Input: part model. Units: mm. Frame: model coordinates. Face numbers are marked on the shaded views. A direction names the side the tool comes from. Give positions to 0.01 mm unless a question says otherwise; leave off trailing zeros. Write each loop counter-clockwise with the first axis right and the second up, starting at its lowest first coordinate (ties: lowest second). Pieces come first, ordered by that corner, then holes. Notation, with made-up numbers: (40.5, 18.25) - (85.5, 18.25) arc R13 ccw to (85.5, 37.25) - close; hole circle Ø4 at (-27.5, 44.25). An arc over 180 degrees is marked (long way). Answer as CSV lines item,"result". Start each with the question number.
from build123d import *

# Parameters (mm, degrees)
BASE_FLANGE1_DEPTH = 15
SKETCH6_R          = 1.64265796
CUT_EXTRUDE1_DEPTH = 0.7


# Sheet-metal steps are written as plain solids
with BuildPart() as part:
    # Sketch1 → Base-Flange1 (new body)
    with BuildSketch(Plane.XY):
        with BuildLine():
            Line((0, 0), (59.3, 0))
            ThreePointArc((59.3, 0), (59.794974747, 0.205025253), (60, 0.7))
            Line((60, 0.7), (60, 73.6))
            ThreePointArc((60, 73.6), (60.410050506, 74.589949494), (61.4, 75))
            Line((61.4, 75), (150, 75))
            Line((150, 75), (150, 74.3))
            Line((150, 74.3), (61.4, 74.3))
            ThreePointArc((61.4, 74.3), (60.905025253, 74.094974747), (60.7, 73.6))
            Line((60.7, 73.6), (60.7, 0.7))
            ThreePointArc((60.7, 0.7), (60.289949494, -0.289949494), (59.3, -0.7))
            Line((59.3, -0.7), (0, -0.7))
            Line((0, -0.7), (0, 0))
        make_face()
    extrude(amount=BASE_FLANGE1_DEPTH)

    # Sketch6 → Cut-Extrude1 (cut)
    with BuildSketch(Plane(origin=(0, 0, 0), x_dir=(1, 0, 0), z_dir=(0, 1, 0))):
        with Locations(Location((15, -7.5, 0), (0, 0, 270))):
            Circle(SKETCH6_R)
        with Locations(Location((45, -7.5, 0), (0, 0, 270))):
            Circle(SKETCH6_R)
    extrude(amount=-CUT_EXTRUDE1_DEPTH, mode=Mode.SUBTRACT)


solid = part.part
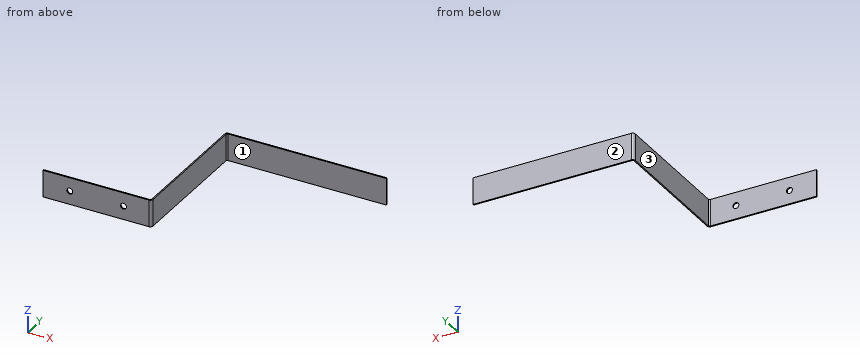
1) Cut plane A-A on z = 7.5. Output: boundary loops of the cut face in (x, y), and give its area (3 significant figures).
2) Material intervals for line 1 (X direction, y = -0.5, z = 7.5); line 2 (X direction, y = -0.2, z = 7.5); line 3 (Y direction, x = 41, z = 12.75), sorted ascending. Write a range as from..to.
3) Reachability of the marked faces 1, 2 and 3 from +Z, -Z, +X, -X, +Y, -Y: full face, straight path, thin tool, end or side. Return the list, or none.
4) Contact query for flat-ended pins moving along their axis: P1, Ø1, axis at x = 113, z = 2.5, coming from the -Y side; P2, Ø7.5, axis at x = 26.5, z = 9.5, coming from the +Y side; P3, Ø2, axis at y = 8, z = 11.5, coming from the +X side. Output: stop coordinate, or through.
5) Cut plane B-B on x = 15. Output: boundary loops of the cut face in (y, z).
6) Cut plane C-C on y = 22. Output: boundary loops of the cut face in (x, z), and give its area (3 significant figures).
Numbers:
1,outline,"(0, -0.7) - (13.36, -0.7) - (13.36, 0) - (0, 0) - close; (16.64, -0.7) - (43.36, -0.7) - (43.36, 0) - (16.64, 0) - close; (46.64, -0.7) - (59.3, -0.7) arc R1.4 ccw to (60.7, 0.7) - (60.7, 73.6) arc R0.7 cw to (61.4, 74.3) - (150, 74.3) - (150, 75) - (61.4, 75) arc R1.4 ccw to (60, 73.6) - (60, 0.7) arc R0.7 cw to (59.3, 0) - (46.64, 0) - close"
1,area,"152 mm²"
2,line 1,"x = 0..13.36, 16.64..43.36, 46.64..60.02"
2,line 2,"x = 0..13.36, 16.64..43.36, 46.64..60.37"
2,line 3,"y = -0.7..0"
3,face 1,"+Z, -Z, +X, -Y"
3,face 2,"+Z, -Z, +X, -X, +Y"
3,face 3,"+Z, -Z, -X, +Y"
4,P1,"stops at y = 74.3"
4,P2,"stops at y = 0"
4,P3,"stops at x = 60.7"
5,outline,"(-0.7, 0) - (0, 0) - (0, 5.86) - (-0.7, 5.86) - close; (-0.7, 9.14) - (0, 9.14) - (0, 15) - (-0.7, 15) - close"
6,outline,"(60, 0) - (60.7, 0) - (60.7, 15) - (60, 15) - close"
6,area,"10.5 mm²"
